Solid Edge part; units mm, degrees
sketch "Sketch1" plane through (0, 0, 0) normal (0, 0, 1) x (1, 0, 0)
  line L0 (-75.298, 50.798) -> (75.298, 50.798)
  line L1 (75.298, 50.798) -> (75.298, -50.798)
  line L2 (75.298, -50.798) -> (-75.298, -50.798)
  line L3 (-75.298, -50.798) -> (-75.298, 50.798)
  dimension "D1" = 75.298
  dimension "D2" = 75.298
extrude "Basiskörper" add sketch "Sketch1" along normal blind 50.8
fillet "Round1" radius 5 4 edges at (75.298, 50.798, 25.4) (75.298, -50.798, 25.4) (-75.298, -50.798, 25.4) (-75.298, 50.798, 25.4)
shell "Thinwall1" thickness 3.798 removed faces 1 at (51.7046, -32.8494, 50.8)
sketch "Sketch2" plane through (0, 0, 3.798) normal (0, 0, 1) x (0, -1, 0)
  circle A0 centre (37, 54.702) radius 5.5
  circle A1 centre (37, -54.298) radius 5.5
  circle A2 centre (-37, -54.298) radius 5.5
  circle A3 centre (-37, 54.702) radius 5.5
  dimension "D1" = 37
extrude "Protrusion1" add sketch "Sketch2" along normal blind 10
hole "Hole1" at (54.702, 37, 13.798) direction (0, 0, -1) diameter 1.5 depth 8 start chamfer 0.6 start chamfer angle 45
hole "Hole2" at (54.702, -37, 13.798) direction (0, 0, -1) diameter 1.5 depth 8 start chamfer 0.6 start chamfer angle 45
hole "Hole3" at (-54.298, 37, 13.798) direction (0, 0, -1) diameter 1.5 depth 8 start chamfer 0.6 start chamfer angle 45
hole "Hole4" at (-54.298, -37, 13.798) direction (0, 0, -1) diameter 1.5 depth 8 start chamfer 0.6 start chamfer angle 45
sketch "Sketch3" plane through (0, 0, 3.798) normal (0, 0, 1) x (0, -1, 0)
  circle A0 centre (44.328, 68.828) radius 5
  circle A1 centre (44.328, -68.828) radius 5
  circle A2 centre (-44.328, -68.828) radius 5
  circle A3 centre (-44.328, 68.828) radius 5
extrude "Protrusion2" add sketch "Sketch3" along normal blind 42.804
hole "Hole5" at (68.828, 44.328, 46.602) direction (0, 0, -1) diameter 4 depth 20 start chamfer 0.4 start chamfer angle 45
hole "Hole6" at (-68.828, -44.328, 46.602) direction (0, 0, -1) diameter 4 depth 20 start chamfer 0.4 start chamfer angle 45
hole "Hole7" at (-68.828, 44.328, 46.602) direction (0, 0, -1) diameter 4 depth 20 start chamfer 0.4 start chamfer angle 45
hole "Hole8" at (68.828, -44.328, 46.602) direction (0, 0, -1) diameter 4 depth 20 start chamfer 0.4 start chamfer angle 45
fillet "Round2" radius 2 8 edges at (71.5, 40.1018, 25.2) (64.6018, 47, 25.2) (71.5, -40.1018, 25.2) (64.6018, -47, 25.2) (-64.6018, 47, 25.2) (-71.5, 40.1018, 25.2) (-71.5, -40.1018, 25.2) (-64.6018, -47, 25.2)
sketch "Sketch4" plane through (0, 0, 0) normal (0, 0, -1) x (1, 0, 0)
  line L0 (-75.298, 39.798) -> (-79.096, 39.798)
  line L1 (-79.096, 39.798) -> (-79.096, -39.798)
  line L2 (-79.096, -39.798) -> (-75.298, -39.798)
  line L3 (-75.298, -39.798) -> (-75.298, 39.798)
  dimension "D1" = 75.298
  dimension "D2" = 79.096
extrude "Protrusion3" add sketch "Sketch4" against normal blind 70.8
sketch "Sketch5" plane through (-70.197, 0, 70.8) normal (0, 0, 1) x (0, -1, 0)
  line L0 (-39.798, -5.101) -> (39.798, -5.101)
  line L1 (39.798, -5.101) -> (39.798, -5.301)
  line L2 (39.798, -5.301) -> (-39.798, -5.301)
  line L3 (-39.798, -5.301) -> (-39.798, -5.101)
  dimension "D1" = 39.798
extrude "Cutout1" cut sketch "Sketch5" against normal blind 20
fillet "VerrundungStänderAussen" radius 1.5 2 edges at (-79.096, -39.798, 35.4) (-79.096, 39.798, 35.4)
hole "Ständer_Löcher_Bohrung" at (-75.298, 32.5, 62.8) direction (-1, 0, 0) diameter 4.5 end up to next
hole "Hole9" at (-75.298, 0, 62.8) direction (-1, 0, 0) diameter 4.5 end up to next
hole "Hole10" at (-75.298, -32.5, 62.8) direction (-1, 0, 0) diameter 4.5 end up to next
fillet "Round3" radius 1.5 2 edges at (-75.498, -39.798, 60.8) (-75.498, 39.798, 60.8)
fillet "VerrundungStänderansatz" radius 1.5 2 edges at (-75.298, -39.798, 25.4) (-75.298, 39.798, 25.4)
sketch "Sketch6" plane through (0, 0, 3.798) normal (0, 0, 1) x (1, 0, 0)
  circle A0 centre (-77.1667, 53.0605) radius 5
  circle A1 centre (77.4871, 52.7469) radius 5
  circle A2 centre (77.9989, -52.0993) radius 5
  circle A3 centre (-76.4405, -53.6001) radius 5
extrude "DruckStabilisatoren" add sketch "Sketch6" against normal blind 3
properties material "ASA"
Geometry check sheet. Reference: the model listing, model coordinates, mm. A direction names the side the tool comes from. Give positions to 0.01 mm unless a question says otherwise; leave off trailing zeros. Order: outer loops, then holes, each group sorted by start corner. A loop starts at its lowest first (then second) coordinate and runs counter-clockwise, first axis right, second up. Notation, with made-up numbers: (56.25, 50) - (87.25, 50) arc R23 ccw to (87.25, 85) - close; hole circle Ø3 at (4.5, 67). An arc over 180 degrees is marked (long way). Answer as a JSON object with one key per item and string values.
(1) Draft check along Y on faces 1 (the cylindrical face through (-54.54, 42.495, 8.728)), 2 (the flat face through (-1, 50.798, 25)), 3 (the flat face through (69, 44, 26.602)), 4 (the flat face through (77, 53, 3.798)). Enter one of: released by +Y, released by -Y, zero draft, split by the parting line, or undercut.
Report:
{"face 1": "undercut", "face 2": "released by +Y", "face 3": "undercut", "face 4": "zero draft"}
(2) Cross-section at C-C (z = 49). Record the cut outline in (x, y), then the cut area to 3 significant figures.
Report:
{"outline": "(-79.1, -38.3) arc R1.5 ccw to (-77.6, -39.8) - (-76.8, -39.8) arc R1.5 cw to (-75.3, -41.3) - (-75.3, -45.8) arc R5 ccw to (-70.3, -50.8) - (70.3, -50.8) arc R5 ccw to (75.3, -45.8) - (75.3, 45.8) arc R5 ccw to (70.3, 50.8) - (-70.3, 50.8) arc R5 ccw to (-75.3, 45.8) - (-75.3, 41.3) arc R1.5 cw to (-76.8, 39.8) - (-77.6, 39.8) arc R1.5 ccw to (-79.1, 38.3) - close; hole (-71.5, -45.8) arc R1.2 ccw to (-70.3, -47) - (70.3, -47) arc R1.2 ccw to (71.5, -45.8) - (71.5, 45.8) arc R1.2 ccw to (70.3, 47) - (-70.3, 47) arc R1.2 ccw to (-71.5, 45.8) - close", "area": "2,140 mm^2"}
(3) Depth check by flat-ended pin: pin 1 Ø0.9 at (x, y) = (54.702, -37) entering from +Z; pin 2 Ø5 at (x, y) = (75.5, 50.5) entering from +Z; pin 3 Ø6 at (x, z) = (9, 44) entering from -Y. Enter the tip coordinate at first touch or a pass-through.
Report:
{"pin 1": "z = 5.8", "pin 2": "z = 50.8", "pin 3": "y = -50.8"}
(4) Cross-section at A-A (z = 62.8). Record the cut outline in (x, y).
Report:
{"outline": "(-79.1, -38.3) arc R1.5 ccw to (-77.6, -39.8) - (-77, -39.8) arc R1.5 ccw to (-75.5, -38.3) - (-75.5, -34.75) - (-79.1, -34.75) - close; (-79.1, -30.25) - (-75.5, -30.25) - (-75.5, -2.25) - (-79.1, -2.25) - close; (-79.1, 2.25) - (-75.5, 2.25) - (-75.5, 30.25) - (-79.1, 30.25) - close; (-79.1, 34.75) - (-75.5, 34.75) - (-75.5, 38.3) arc R1.5 ccw to (-77, 39.8) - (-77.6, 39.8) arc R1.5 ccw to (-79.1, 38.3) - close"}
(5) Cross-section at B-B (y = 0). Record the cut outline in (x, z), then the cut area to 3 significant figures.
Report:
{"outline": "(-79.1, 0) - (75.3, 0) - (75.3, 50.8) - (71.5, 50.8) - (71.5, 3.8) - (-71.5, 3.8) - (-71.5, 50.8) - (-75.5, 50.8) - (-75.5, 60.55) - (-79.1, 60.55) - close; (-79.1, 65.05) - (-75.5, 65.05) - (-75.5, 70.8) - (-79.1, 70.8) - close", "area": "1,180 mm^2"}
(6) Tool access check on faces 5 (the flat face through (77, 53, 0.798)), 6 (the flat face through (1, -47, 27)), 7 (the cylindrical face through (-77.272, 0.099, 65.048)). Record the directions out of +Z, -Z, +X, -X, +Y, -Y that give a thin tool (end or side, any length) a straight path to the whole face; none if there is none.
Report:
{"face 5": "-Z, +X, +Y", "face 6": "+Z", "face 7": "+X, -X"}
(7) Cross-section at D-D (x = -19). Record the cut outline in (y, z), then the cut area to 3 significant figures.
Report:
{"outline": "(-50.8, 0) - (50.8, 0) - (50.8, 50.8) - (47, 50.8) - (47, 3.8) - (-47, 3.8) - (-47, 50.8) - (-50.8, 50.8) - close", "area": "743 mm^2"}
(8) Material ranges on line 1 (X direction, y = -37, z = 9.75); line 2 (X direction, y = -1.5, z = 24); line 3 (Y direction, x = 26.5, z = 29), recorded low to high.
Report:
{"line 1": "-79.1 to -71.5, -59.8 to -55.05, -53.55 to -48.8, 49.2 to 53.95, 55.45 to 60.2, 71.5 to 75.3", "line 2": "-79.1 to -71.5, 71.5 to 75.3", "line 3": "-50.8 to -47, 47 to 50.8"}
